Read the model definition and answer for the solid it produces. Units are mm, in the model's axes. Face numbers are marked on the shaded views. Give positions to 0.01 mm unless a question says otherwise; leave off trailing zeros. Loops run counter-clockwise (first coordinate to the right, second up) from the corner with the lowest first, then second, coordinate; pieces in that order, holes last. Notation, with made-up numbers: (57.25, -37.75) - (80.25, -37.75) arc R25 ccw to (80.25, 0.25) - close; hole circle Ø11 at (83.5, 54). An arc over 180 degrees is marked (long way). Write item = value, one per line.
```python
from build123d import *

# Parameters (mm, degrees)
SKETCH036_W          = 31.5
SKETCH036_H          = 20
PAD022_DEPTH         = 51
PAD022_DEPTH_BACK    = 48
THICKNESS006_T       = 1.5
POCKET008_DEPTH      = 49.501
SKETCH039_W          = 11.02125
SKETCH039_H          = 25.4
SKETCH039_W_2        = 5
POCKET010_DEPTH      = 5
SKETCH040_W          = 6.35
SKETCH040_H          = 15.173466
POCKET011_DEPTH      = 17.251
POCKET011_DEPTH_BACK = 17.251
SKETCH044_R          = 3.25
SKETCH044_W          = 25
SKETCH044_H          = 13.75
POCKET013_DEPTH      = 11.501
CHAMFER006_SIZE      = 1.25
SKETCH049_W          = 36.888542
SKETCH049_H          = 25.404094
SKETCH049_W_2        = 33
SKETCH049_H_2        = 21.5
POCKET015_DEPTH      = 2.001
FILLET008_R          = 1


with BuildPart() as part:
    # Sketch036 → Pad022 (new body, two sides)
    with BuildSketch(Plane.XY) as pad022_sk:
        Rectangle(SKETCH036_W, SKETCH036_H)
    extrude(amount=PAD022_DEPTH)
    extrude(pad022_sk.sketch, amount=-PAD022_DEPTH_BACK)

    # Thickness006
    thickness006_openings = [part.faces().sort_by_distance(p)[0] for p in [
        (0, 0, 51),
    ]]
    offset(amount=THICKNESS006_T, openings=thickness006_openings)

    # Sketch037 → Pocket008 (cut, through all)
    with BuildSketch(Plane.XY):
        Polygon((-4.25, 9), (4.25, 9), (4.25, 7.25), (2.5, 5.5), (-2.5, 5.5), (-4.25, 7.25), align=None)
    extrude(amount=-POCKET008_DEPTH, mode=Mode.SUBTRACT)

    # Sketch039 → Pocket010 (cut)
    with BuildSketch(Plane.XZ.offset(7)):
        with Locations((-21.146455, 0)):
            Rectangle(SKETCH039_W, SKETCH039_H)
        with Locations((-6.045277, 0)):
            Rectangle(SKETCH039_W_2, SKETCH039_H)
        with Locations((6.045277, 0)):
            Rectangle(SKETCH039_W_2, SKETCH039_H)
        with Locations((21.146455, 0)):
            Rectangle(SKETCH039_W, SKETCH039_H)
    extrude(amount=POCKET010_DEPTH, mode=Mode.SUBTRACT)

    # Sketch040 → Pocket011 (cut, two sides)
    with BuildSketch(Plane.YZ) as pocket011_sk:
        with Locations((-6.325, 43.836733)):
            Rectangle(SKETCH040_W, SKETCH040_H)
    extrude(amount=-POCKET011_DEPTH, mode=Mode.SUBTRACT)
    extrude(pocket011_sk.sketch, amount=POCKET011_DEPTH_BACK, mode=Mode.SUBTRACT)

    # Sketch044 → Pocket013 (cut, through all)
    with BuildSketch(Plane.XZ):
        with Locations((-5.08, 17)):
            Circle(SKETCH044_R)
        with Locations((5.08, 17)):
            Circle(SKETCH044_R)
        with Locations((0, 37.625)):
            Rectangle(SKETCH044_W, SKETCH044_H)
    extrude(amount=-POCKET013_DEPTH, mode=Mode.SUBTRACT)

    # Chamfer006
    chamfer006_edges = [part.edges().sort_by_distance(p)[0] for p in [
        (1.83, 11.5, 17),
        (-8.33, 11.5, 17),
    ]]
    chamfer(chamfer006_edges, length=CHAMFER006_SIZE)

    # Sketch049 → Pocket015 (cut, through all)
    with BuildSketch(Plane.XY.offset(49)):
        Rectangle(SKETCH049_W, SKETCH049_H)
        Rectangle(SKETCH049_W_2, SKETCH049_H_2, mode=Mode.SUBTRACT)
    extrude(amount=POCKET015_DEPTH, mode=Mode.SUBTRACT)

    # Fillet008
    fillet008_edges = [part.edges().sort_by_distance(p)[0] for p in [
        (-16.5, 10.75, 50),
        (-16.5, -10.75, 50),
        (16.5, -10.75, 50),
        (16.5, 10.75, 50),
    ]]
    fillet(fillet008_edges, radius=FILLET008_R)


solid = part.part
```
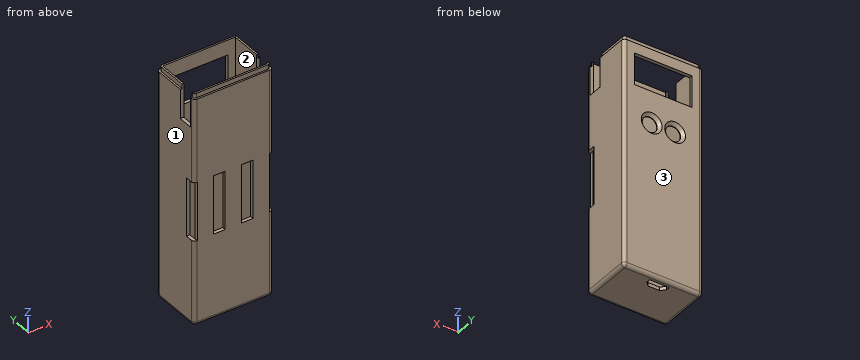
1) A cutting plane is placed at C-C on x = 11. Determine the outline of the cut face in (y, z), then the cut area to 3 significant figures.
Output:
outline = (-11.5, -48) arc R1.5 ccw to (-10, -49.5) - (10, -49.5) arc R1.5 ccw to (11.5, -48) - (11.5, 30.75) - (10, 30.75) - (10, -48) - (-10, -48) - (-10, 51) - (-10.75, 51) - (-10.75, 49) - (-11.5, 49) - close; (10, 44.5) - (11.5, 44.5) - (11.5, 49) - (10.75, 49) - (10.75, 51) - (10, 51) - close
area = 307 mm²
2) A cutting plane is placed at B-B on y = -8. Determine the outline of the cut face in (x, z).
Output:
outline = (-17.25, -48) arc R1.5 ccw to (-15.75, -49.5) - (15.75, -49.5) arc R1.5 ccw to (17.25, -48) - (17.25, -12.7) - (15.75, -12.7) - (15.75, -48) - (-15.75, -48) - (-15.75, -12.7) - (-17.25, -12.7) - close; (-17.25, 12.7) - (-15.75, 12.7) - (-15.75, 36.25) - (-17.25, 36.25) - close; (15.75, 12.7) - (17.25, 12.7) - (17.25, 36.25) - (15.75, 36.25) - close
3) The mould has two halves that part along Y. Classify the marked faces 1, 2 and 3: pulls with the +Y half, pulls with the -Y half, needs draft (parallel to the pull), parting line crosses it, or undercut.
Output:
face_1 = needs draft
face_2 = undercut
face_3 = pulls with the +Y half
4) A cutting plane is placed at D-D on z = -15. Determine the outline of the cut face in (x, y), then the cut area to 3 significant figures.
Output:
outline = (-17.25, -10) arc R1.5 ccw to (-15.75, -11.5) - (15.75, -11.5) arc R1.5 ccw to (17.25, -10) - (17.25, 10) arc R1.5 ccw to (15.75, 11.5) - (-15.75, 11.5) arc R1.5 ccw to (-17.25, 10) - close; hole (-15.75, -10) - (15.75, -10) - (15.75, 10) - (-15.75, 10) - close
area = 162 mm²
5) A cutting plane is placed at A-A on z = 17. Determine the outline of the cut face in (x, y), then the cut area to 3 significant figures.
Output:
outline = (-17.25, -10) arc R1.5 ccw to (-15.75, -11.5) - (15.75, -11.5) arc R1.5 ccw to (17.25, -10) - (17.25, 10) arc R1.5 ccw to (15.75, 11.5) - (9.58, 11.5) - (8.33, 10.25) - (8.33, 10) - (15.75, 10) - (15.75, -10) - (-15.75, -10) - (-15.75, 10) - (-8.33, 10) - (-8.33, 10.25) - (-9.58, 11.5) - (-15.75, 11.5) arc R1.5 ccw to (-17.25, 10) - close; (-1.83, 10) - (1.83, 10) - (1.83, 10.25) - (0.58, 11.5) - (-0.58, 11.5) - (-1.83, 10.25) - close
area = 139 mm²
6) Each of these flat-tipped pins is pushed along its axis until it touches: P1, Ø1.2, axis at x = -1, z = -49, coming from the -Y side; P2, Ø3, axis at x = -5, y = -4, coming from the +Z side; P3, Ø0.8, axis at x = 17, y = -10, coming from the -Z side. Where does it stop, or does it pass through?
Output:
P1 = -11.45
P2 = -48
P3 = -49.24
7) Find the intervals of material crossed by probe 1 along Z at (x, y) = (-5.08, 10.1); probe 2 along Y at (x, z) = (-14, 38); probe 3 along X at (y, z) = (9, 46), in increasing order.
Output:
probe_1 = -49.5 to 13.75, 20.25 to 30.75, 44.5 to 51
probe_2 = -11.5 to -10, 10 to 11.5
probe_3 = -17.25 to -15.75, 15.75 to 17.25
